Answer from the drawing. Dimensions are ordinates in mm from the lowest x, y and z of the part. Coordinates: 2 decimals unless noted, no trailing zeros. Loops run counter-clockwise (first coordinate to the right, second up) from the corner with the lowest first, then second, coordinate; pieces in that order, holes last. Notation, with made-up numbers: M -39.5,47 L 14.5,47 A8 ccw 14.5,52 Z; hole C 51,86.25 d5. An arc over 180 degrees is marked long. One line per item, written item: value. Start each with the question number.
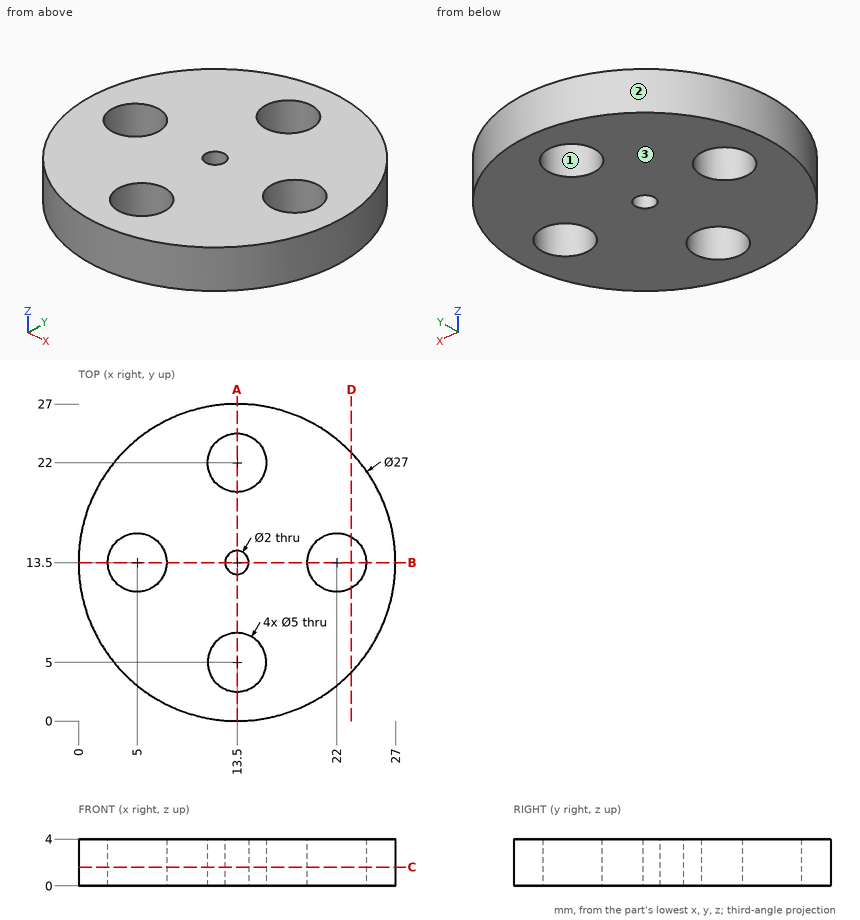
1) Consider line 1 along Y through (x, z) = (13.5, 1.9); line 2 along Y through (x, z) = (14.25, 2.4); line 3 along X through (y, z) = (12, 3.7). Determine where each line is inside the solid, lowest interval first.
2) Section D-D (x = 23.25) is taken. Determine the outline of the cut face in (y, z).
3) Section C-C (z = 1.6) is taken. Determine the outline of the cut face in (x, y), then the cut area to 3 significant figures.
4) Flat-ended cylindrical pins translate along their axes: pin 1 (2 mm diameter, centred on x = 21, z = 3, fed in from -Y); pin 2 (1.5 mm diameter, centred on x = 14.5, z = 2.5, fed in from -Y). Find the tip coordinate at first contact, or state that the pin passes through.
5) For a pull along Y with two mould halves and no side action, classify the marked faces 1, 2 and 3 as released by +Y, released by -Y, zero draft, split by the parting line, or undercut.
6) Section A-A (x = 13.5) is taken. Determine the outline of the cut face in (y, z), then the cut area to 3 significant figures.
Results found:
1. line 1: y = 0 to 2.5, 7.5 to 12.5, 14.5 to 19.5, 24.5 to 27
1. line 2: y = 0.02 to 2.62, 7.38 to 12.84, 14.16 to 19.62, 24.38 to 26.98
1. line 3: x = 0.08 to 3, 7 to 20, 24 to 26.92
2. outline: M 4.16,0 L 11.33,0 L 11.33,4 L 4.16,4 Z; M 15.67,0 L 22.84,0 L 22.84,4 L 15.67,4 Z
3. outline: C 13.5,13.5 d27; hole C 5,13.5 d5; hole C 13.5,5 d5; hole C 13.5,22 d5; hole C 13.5,13.5 d2; hole C 22,13.5 d5
3. area: 491 mm²
4. pin 1: stops at y = 1.67
4. pin 2: stops at y = 0
5. face 1: undercut
5. face 2: split by the parting line
5. face 3: zero draft
6. outline: M 0,0 L 2.5,0 L 2.5,4 L 0,4 Z; M 7.5,0 L 12.5,0 L 12.5,4 L 7.5,4 Z; M 14.5,0 L 19.5,0 L 19.5,4 L 14.5,4 Z; M 24.5,0 L 27,0 L 27,4 L 24.5,4 Z
6. area: 60.0 mm²
